```python
from build123d import *

# Parameters (mm, degrees)
SKETCH_1_W           = 47
SKETCH_1_H           = 42.665281763
SKETCH_1_R           = 2.5
EXTRUDE_1_DEPTH      = 5
SKETCH_2_W           = 6
SKETCH_2_H           = 42.665281763
SKETCH_2_W_2         = 47
SKETCH_2_H_2         = 2
EXTRUDE_2_DEPTH      = 33
SKETCH_3_W           = 40.665281763
SKETCH_3_H           = 33
EXTRUDE_3_DEPTH      = 6
SKETCH_4_R           = 6.5
CUT_EXTRUDE_2_DEPTH  = 7
CHAMFER_1_SIZE       = 3
CUT_EXTRUDE_8_DEPTH  = 25
SKETCH_7_W           = 20.5
SKETCH_7_H           = 8
CUT_EXTRUDE_9_DEPTH  = 10
SKETCH_8_R           = 6.5
EXTRUDE_4_DEPTH      = 5
FILLET_4_R           = 2
SKETCH_9_W           = 11
SKETCH_9_H           = 7.412058926
EXTRUDE_5_DEPTH      = 25
FILLET_5_R           = 10
CUT_EXTRUDE_10_DEPTH = 4


with BuildPart() as part:
    # 草图1 → 凸台-拉伸1 (new body)
    with BuildSketch(Plane(origin=(0, 0, 0), x_dir=(1, 0, 0), z_dir=(0, 1, 0))):
        with Locations((0, 8.371925414)):
            Rectangle(SKETCH_1_W, SKETCH_1_H)
        with Locations((19, -8.15756763)):
            Circle(SKETCH_1_R, mode=Mode.SUBTRACT)
        with Locations((-19, -8.15756763)):
            Circle(SKETCH_1_R, mode=Mode.SUBTRACT)
        with Locations((19, 21.84243237)):
            Circle(SKETCH_1_R, mode=Mode.SUBTRACT)
        with Locations((-19, 21.84243237)):
            Circle(SKETCH_1_R, mode=Mode.SUBTRACT)
    extrude(amount=EXTRUDE_1_DEPTH)

    # 草图2 → 凸台-拉伸2 (add)
    with BuildSketch(Plane(origin=(0, 5, 0), x_dir=(1, 0, 0), z_dir=(0, 1, 0))):
        with Locations((0, 8.371925414)):
            Rectangle(SKETCH_2_W, SKETCH_2_H)
        with Locations((0, 28.704566295)):
            Rectangle(SKETCH_2_W_2, SKETCH_2_H_2)
    extrude(amount=EXTRUDE_2_DEPTH)

    # 草图3 → 凸台-拉伸3 (add)
    with BuildSketch(Plane.ZY.offset(3)):
        with Locations((-7.371925414, 21.5)):
            Rectangle(SKETCH_3_W, SKETCH_3_H)
        with Locations((-7.371925414, 21.5)):
            Rectangle(SKETCH_3_W, SKETCH_3_H)
        with Locations((-7.371925414, 21.5)):
            Rectangle(SKETCH_3_W, SKETCH_3_H)
        with Locations((-7.371925414, 21.5)):
            Rectangle(SKETCH_3_W, SKETCH_3_H)
        with Locations((-7.371925414, 21.5)):
            Rectangle(SKETCH_3_W, SKETCH_3_H)
        with Locations((-7.371925414, 21.5)):
            Rectangle(SKETCH_3_W, SKETCH_3_H)
        with Locations((-7.371925414, 21.5)):
            Rectangle(SKETCH_3_W, SKETCH_3_H)
        with Locations((-7.371925414, 21.5)):
            Rectangle(SKETCH_3_W, SKETCH_3_H)
    extrude(amount=-EXTRUDE_3_DEPTH)

    # 草图4 → 切除-拉伸2 (cut)
    with BuildSketch(Plane(origin=(-3, 2.117173295, 0), x_dir=(0, 0, 1), z_dir=(-1, 0, 0))):
        with Locations((-7.289458503, 20.878429676)):
            Circle(SKETCH_4_R)
    extrude(amount=-CUT_EXTRUDE_2_DEPTH, mode=Mode.SUBTRACT)

    # 倒角1
    chamfer_1_edges = [part.edges().sort_by_distance(p)[0] for p in [
        (23.5, 38, -28.704566295),
        (-23.5, 38, -28.704566295),
    ]]
    chamfer(chamfer_1_edges, length=CHAMFER_1_SIZE)

    # 草图6 → 切除-拉伸8 (cut)
    with BuildSketch(Plane(origin=(0, 38, 0), x_dir=(1, 0, 0), z_dir=(0, 1, 0))):
        Polygon((-26.394551402, 22.292507369), (-3, 22.292507369), (-3, 27.704566295), (-20.5, 27.704566295), (-20.5, 29.704566295), (20.5, 29.704566295), (20.5, 27.704566295), (3, 27.704566295), (3, 22.292507369), (28.987300096, 22.292507369), (28.987300096, 31.415661045), (-26.394551402, 31.415661045), align=None)
        Polygon((-3, 27.704566295), (-3, 22.292507369), (3, 22.292507369), (3, 27.704566295), (20.5, 27.704566295), (20.5, 29.704566295), (-20.5, 29.704566295), (-20.5, 27.704566295), align=None)
    extrude(amount=-CUT_EXTRUDE_8_DEPTH, mode=Mode.SUBTRACT)

    # 草图7 → 切除-拉伸9 (cut)
    with BuildSketch(Plane.XY.offset(-27.704566295)):
        with Locations((13.25, 9)):
            Rectangle(SKETCH_7_W, SKETCH_7_H)
    extrude(amount=-CUT_EXTRUDE_9_DEPTH, mode=Mode.SUBTRACT)

    # 草图8 → 凸台-拉伸4 (add)
    with BuildSketch(Plane.ZY.offset(3)):
        Polygon((12.960715468, 38), (-22.292507369, 38), (-22.292507369, 13), (-27.704566295, 13), (-27.704566295, 5), (12.960715468, 5), align=None)
        with Locations((-7.289458503, 22.995602971)):
            Circle(SKETCH_8_R, mode=Mode.SUBTRACT)
    extrude(amount=EXTRUDE_4_DEPTH)

    # 圆角4
    fillet_4_edges = [part.edges().sort_by_distance(p)[0] for p in [
        (-8, 9, -27.704566295),
    ]]
    fillet(fillet_4_edges, radius=FILLET_4_R)

    # 草图9 → 凸台-拉伸5 (add)
    with BuildSketch(Plane(origin=(0, 13, 0), x_dir=(1, 0, 0), z_dir=(0, 1, 0))):
        with Locations((-2.5, 25.998536832)):
            Rectangle(SKETCH_9_W, SKETCH_9_H)
    extrude(amount=EXTRUDE_5_DEPTH)

    # 圆角5
    fillet_5_edges = [part.edges().sort_by_distance(p)[0] for p in [
        (-2.5, 38, -29.704566295),
        (-2.5, 38, 12.960715468),
    ]]
    fillet(fillet_5_edges, radius=FILLET_5_R)

    # 草图10 → 切除-拉伸10 (cut)
    with BuildSketch(Plane(origin=(0, 0, -29.704566295), x_dir=(-1, 0, 0), z_dir=(0, 0, -1))):
        with BuildLine():
            ThreePointArc((18.603175919, 9), (16.603175919, 11), (14.603175919, 9))
            Line((14.603175919, 9), (18.603175919, 9))
        make_face()
        with BuildLine():
            Line((18.603175919, 9), (14.603175919, 9))
            ThreePointArc((14.603175919, 9), (16.603175919, 7), (18.603175919, 9))
        make_face()
        with BuildLine():
            ThreePointArc((18.603175919, 9), (16.603175919, 11), (14.603175919, 9))
            Line((14.603175919, 9), (18.603175919, 9))
        make_face()
        with BuildLine():
            Line((18.603175919, 9), (14.603175919, 9))
            ThreePointArc((14.603175919, 9), (16.603175919, 7), (18.603175919, 9))
        make_face()
        with BuildLine():
            ThreePointArc((4.5, 14.309411668), (3.914213562, 15.723625231), (2.5, 16.309411668))
            Line((2.5, 16.309411668), (2.5, 12.309411668))
            ThreePointArc((2.5, 12.309411668), (3.914213562, 12.895198106), (4.5, 14.309411668))
        make_face()
        with BuildLine():
            Line((2.5, 12.309411668), (2.5, 16.309411668))
            ThreePointArc((2.5, 16.309411668), (0.5, 14.309411668), (2.5, 12.309411668))
        make_face()
        with BuildLine():
            ThreePointArc((4.5, 14.309411668), (3.914213562, 15.723625231), (2.5, 16.309411668))
            Line((2.5, 16.309411668), (2.5, 12.309411668))
            ThreePointArc((2.5, 12.309411668), (3.914213562, 12.895198106), (4.5, 14.309411668))
        make_face()
        with BuildLine():
            Line((2.5, 12.309411668), (2.5, 16.309411668))
            ThreePointArc((2.5, 16.309411668), (0.5, 14.309411668), (2.5, 12.309411668))
        make_face()
    extrude(amount=-CUT_EXTRUDE_10_DEPTH, mode=Mode.SUBTRACT)


solid = part.part
```
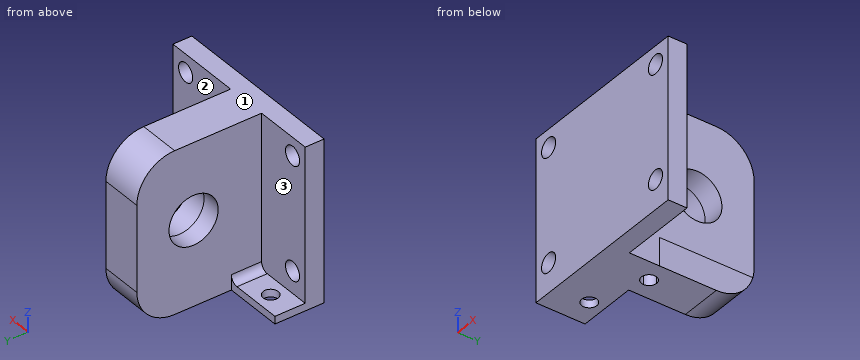
For this review, take the finished solid that the model builds, in its own axes (mm). Face numbers are marked on the shaded views. A direction names the side the tool comes from. Give positions to 0.01 mm unless a question says otherwise; leave off trailing zeros. Order: outer loops, then holes, each group sorted by start corner. A loop starts at its lowest first (then second) coordinate and runs counter-clockwise, first axis right, second up.
1) Take a section at A-A (y = 9). Give the boundary of the cut face in (x, z), then the cut area to 3 significant figures.
2) Insertion check: pin 1 (6 mm diameter, centred on y = 25, z = -24, fed in from +X); pin 2 (3 mm diameter, centred on x = -2, y = 14, fed in from -Z); pin 3 (10 mm diameter, centred on x = 5, z = -25, fed in from +Y); pin 4 (4.5 mm diameter, centred on x = -18.5, z = -5.5, fed in from +Y). Each pin has a flat end and moves straight along its axis. Give the tip position at first contact, or say it passes through.
3) Wall thickness on line 1 (Z direction, x = -19, y = 1.25); line 2 (X direction, y = 9, z = -29); line 3 (X direction, y = 29.5, z = -25.5): over which ranges is each line inside the solid? List them lowest first.
4) Take a section at B-B (x = 19). Give the boundary of the cut face in (y, z).
5) Take a section at C-C (z = -23.5). Give the boundary of the cut face in (x, y).
6) Take a section at D-D (y = 26.5). Give the boundary of the cut face in (x, z), then the cut area to 3 significant figures.
7) For the marked faces 1, 2 and 3, list the 3-axis set-ups (+Z, -Z, +X, -X, +Y, -Y) from which the entire face can be reached by the end or side of a thin tool; tool diameter is ignored.
Derived:
1. outline: (-23.5, -29.7) - (-18.6, -29.7) - (-18.6, -27.7) - (-23.5, -27.7) - close; (-14.6, -29.7) - (3, -29.7) - (3, 12.96) - (-8, 12.96) - (-8, -25.7) arc R2 cw to (-10, -27.7) - (-14.6, -27.7) - close
1. area: 493 mm2
2. pin 1: stops at x = 3
2. pin 2: stops at z = -29.7
2. pin 3: stops at y = 37.97
2. pin 4: stops at y = 5
3. line 1: z = -29.7 to -24.34, -19.34 to 5.66, 10.66 to 12.96
3. line 2: x = -23.5 to -18.6, -14.6 to 3
3. line 3: x = -8 to 3
4. outline: (0, -29.7) - (5, -29.7) - (5, -24.34) - (0, -24.34) - close; (0, -19.34) - (5, -19.34) - (5, 5.66) - (0, 5.66) - close; (0, 10.66) - (5, 10.66) - (5, 12.96) - (0, 12.96) - close
5. outline: (-23.5, 0) - (-20.87, 0) - (-20.87, 5) - (-23.5, 5) - close; (-17.13, 0) - (17.13, 0) - (17.13, 5) - (3, 5) - (3, 37.25) - (-8, 37.25) - (-8, 5) - (-17.13, 5) - close; (20.87, 0) - (23.5, 0) - (23.5, 5) - (20.87, 5) - close
6. outline: (-8, -29.7) - (3, -29.7) - (3, -12.76) - (-8, -12.76) - close; (-8, -1.82) - (3, -1.82) - (3, 12.96) - (-8, 12.96) - close
6. area: 349 mm2
7. face 1: +Z, +X, -X, +Y, -Y
7. face 2: +Z, -Z, +X, +Y
7. face 3: +Z, -X, +Y
